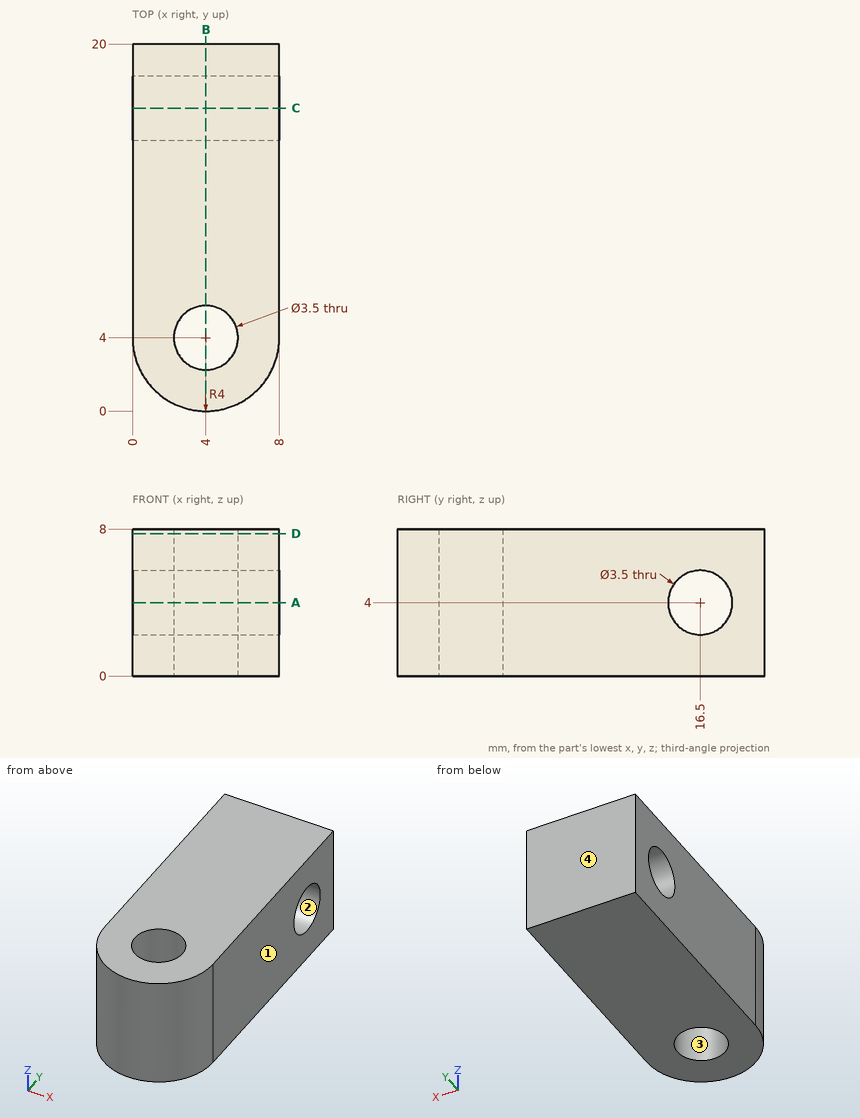
Print and shaded views of the part. All mm, measured from the part's lowest x, y and z. Coordinates: 2 decimals unless noted, no trailing zeros. Order: outer loops, then holes, each group sorted by start corner. A loop starts at its lowest first (then second) coordinate and runs counter-clockwise, first axis right, second up. Notation, with made-up numbers: M -36,27.25 L 4,27.25 A9 ccw 4,37.25 Z; hole C -12.5,52.25 d5. An arc over 180 degrees is marked long. Answer as CSV lines item,"result".
1) Cut at B-B (x = 4). List the corners of the cut face in (y, z).
Verdict:
outline,"M 0,0 L 2.25,0 L 2.25,8 L 0,8 Z; M 5.75,0 L 20,0 L 20,8 L 5.75,8 Z; hole C 16.5,4 d3.5"
2) Flat gauge pins, fed straight in: P1, Ø3, axis at x = 4, y = 4, coming from the -Z side (3 decimals); P2, Ø4, axis at y = 16.5, z = 4, coming from the +X side. Where does each tip first touch, or does it go through?
Verdict:
P1,"through"
P2,"x = 8"
3) Mould opens along Y. For the marked faces 1, 2, 3 and 4 say: released by +Y, released by -Y, zero draft, split by the parting line, or undercut.
Verdict:
face 1,"zero draft"
face 2,"undercut"
face 3,"undercut"
face 4,"released by +Y"
4) Drill centre lines: L1, parallel to Z at x = 5.5, y = 16.5; L2, parallel to Y at x = 4, z = 1.5; L3, parallel to X at y = 3.5, z = 2.75. Where is each one in solid material? Low to high. Write a range as from..to.
Verdict:
L1,"0..2.25, 5.75..8"
L2,"0..2.25, 5.75..20"
L3,"0.03..2.32, 5.68..7.97"
5) Cut at A-A (z = 4). List the corners of the cut face in (x, y).
Verdict:
outline,"M 0,4 A4 ccw 8,4 L 8,14.75 L 0,14.75 Z; M 0,18.25 L 8,18.25 L 8,20 L 0,20 Z; hole C 4,4 d3.5"
6) Cut at D-D (z = 7.75). List the corners of the cut face in (x, y), then the cut area to 3 significant figures.
Verdict:
outline,"M 0,4 A4 ccw 8,4 L 8,20 L 0,20 Z; hole C 4,4 d3.5"
area,"144 mm2"
7) Cut at C-C (y = 16.5). List the corners of the cut face in (x, z).
Verdict:
outline,"M 0,0 L 8,0 L 8,2.25 L 0,2.25 Z; M 0,5.75 L 8,5.75 L 8,8 L 0,8 Z"
